```python
from build123d import *

# Parameters (mm, degrees)
BOSS_EXTRUDE1_DEPTH            = 294.55
FILLET1_R                      = 1.5875
CUT_EXTRUDE1_DEPTH             = 306.043611636
CUT_EXTRUDE1_DEPTH_BACK        = 306.043611636
F_7_9_7_9_DIAMETER_HOLE2_D     = 7.9
F_7_9_7_9_DIAMETER_HOLE2_DEPTH = 15
F_7_9_7_9_DIAMETER_HOLE2_TIP   = 2.373399445
CUT_EXTRUDE3_DEPTH             = 306.043611636
CUT_EXTRUDE3_DEPTH_BACK        = 306.043611636
SKETCH9_W                      = 91.05
SKETCH9_H                      = 25
SKETCH9_H_2                    = 5.6275
SKETCH9_H_3                    = 1.5875
FILLET2_R                      = 3.175


with BuildPart() as part:
    # Sketch1 → Boss-Extrude1 (new, symmetric)
    with BuildSketch(Plane.XY):
        Polygon((0, 77), (0, 0), (4.05, 0), (4.05, 9.525), (19.05, 9.525), (19.05, 70), (4.05, 70), (4.05, 77), align=None)
    extrude(amount=BOSS_EXTRUDE1_DEPTH, both=True)

    # Fillet1
    fillet1_edges = [part.edges().sort_by_distance(p)[0] for p in [
        (0, 0, 0),
        (0, 77, 0),
    ]]
    fillet(fillet1_edges, radius=FILLET1_R)

    # Sketch2 → Cut-Extrude1 (cut, two sides: drawn at the far end of the back side and taken through both)
    with BuildSketch(Plane(origin=(0, 77, 0), x_dir=(1, 0, 0), z_dir=(0, 1, 0)).offset(-CUT_EXTRUDE1_DEPTH_BACK)):
        Polygon((0, 294.55), (19.05, 275.5), (19.05, 294.55), align=None)
        Polygon((19.05, -275.5), (19.05, -294.55), (0, -294.55), align=None)
    extrude(amount=CUT_EXTRUDE1_DEPTH + CUT_EXTRUDE1_DEPTH_BACK, mode=Mode.SUBTRACT)

    # Ø7.9 (7.9) Diameter Hole2
    with Locations(Plane.XZ.offset(-9.525)):
        with Locations((11.55, -104.55), (11.55, 104.55)):
            Hole(F_7_9_7_9_DIAMETER_HOLE2_D / 2, depth=F_7_9_7_9_DIAMETER_HOLE2_DEPTH)
            with Locations((0, 0, -(F_7_9_7_9_DIAMETER_HOLE2_DEPTH + F_7_9_7_9_DIAMETER_HOLE2_TIP / 2))):  # 118° drill point
                Cone(0, F_7_9_7_9_DIAMETER_HOLE2_D / 2, F_7_9_7_9_DIAMETER_HOLE2_TIP, mode=Mode.SUBTRACT)

    # Sketch9 → Cut-Extrude3 (cut, two sides: drawn at the far end of the back side and taken through both)
    with BuildSketch(Plane.ZY.offset(-CUT_EXTRUDE3_DEPTH_BACK)):
        with Locations((0, 19.715)):
            Rectangle(SKETCH9_W, SKETCH9_H)
        with Locations((0, 4.40125)):
            Rectangle(SKETCH9_W, SKETCH9_H_2)
        with Locations((0, 0.79375)):
            Rectangle(SKETCH9_W, SKETCH9_H_3)
    extrude(amount=CUT_EXTRUDE3_DEPTH + CUT_EXTRUDE3_DEPTH_BACK, mode=Mode.SUBTRACT)

    # Fillet2
    fillet2_edges = [part.edges().sort_by_distance(p)[0] for p in [
        (9.525, 32.215, 45.525),
        (9.525, 32.215, -45.525),
    ]]
    fillet(fillet2_edges, radius=FILLET2_R)


solid = part.part
```
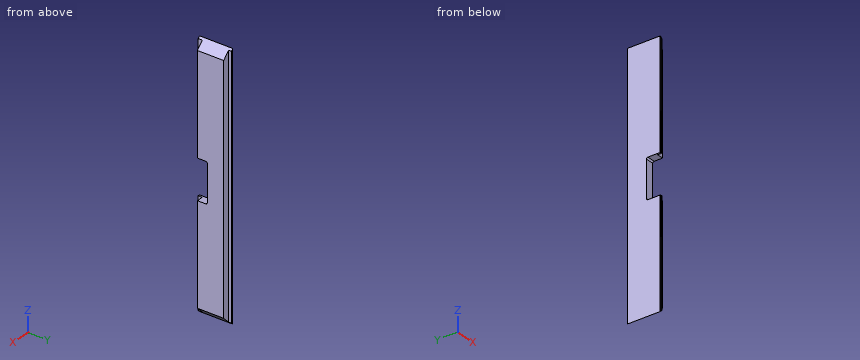
Work out the finished part from the listing and answer in its coordinate system (mm). Round coordinates to 2 decimals unless told otherwise and drop trailing zeros. Write each loop counter-clockwise with the first axis right and the second up, starting at its lowest first coordinate (ties: lowest second). Pieces come first, ordered by that corner, then holes.
1) Consider probe 1 along X at (y, z) = (20.75, 104.55); probe 2 along X at (y, z) = (14, -104); probe 3 along Z at (x, y) = (11.55, 14.5) (3 decimals). Determine where each line is inside the solid, lowest interval first.
2) A cutting plane is placed at A-A on y = 15. Determine the outline of the cut face in (x, z) (3 decimals).
3) Flat-ended cylindrical pins translate along their axes: P1, Ø1, axis at x = 6.5, y = 57.5, coming from the -Z side; P2, Ø6, axis at x = 7.5, y = 25, coming from the -Z side; P3, Ø4.5, axis at x = 9.5, z = -145.5, coming from the -Y side (3 decimals). Find the tip coordinate at first contact, or state that the pin passes through.
4) A cutting plane is placed at C-C on y = 53. Determine the outline of the cut face in (x, z), and give its area (3 significant figures).
Entries:
1. probe 1: x = 0 to 7.6, 15.5 to 19.05
1. probe 2: x = 0 to 7.64, 15.46 to 19.05
1. probe 3: z = -283 to -108.5, -100.6 to -45.525, 45.525 to 100.6, 108.5 to 283
2. outline: (0, -294.55) - (19.05, -275.5) - (19.05, -45.525) - (0, -45.525) - close; (0, 45.525) - (19.05, 45.525) - (19.05, 275.5) - (0, 294.55) - close; hole circle Ø7.9 at (11.55, -104.55); hole circle Ø7.9 at (11.55, 104.55)
3. P1: stops at z = -288.55
3. P2: stops at z = -290.05
3. P3: stops at y = 9.525
4. outline: (0, -294.55) - (19.05, -275.5) - (19.05, 275.5) - (0, 294.55) - close
4. area: 10,900 mm2
